from build123d import *

# Parameters (mm, degrees)
SKETCH1_W           = 22
SKETCH1_H           = 50
BOSS_EXTRUDE1_DEPTH = 4.25


with BuildPart() as part:
    # Sketch1 → Boss-Extrude1 (new body, symmetric)
    with BuildSketch(Plane.XY):
        with BuildLine():
            Line((-498.569276331, 84.968707483), (501.430723669, 84.968707483))
            Line((501.430723669, 84.968707483), (501.430723669, 62.328707483))
            ThreePointArc((501.430723669, 62.328707483), (498.250723669, 59.148707483), (501.430723669, 55.968707483))
            Line((501.430723669, 55.968707483), (551.430723669, 55.968707483))
            Line((551.430723669, 55.968707483), (551.430723669, -53.031292517))
            Line((551.430723669, -53.031292517), (501.430723669, -53.031292517))
            ThreePointArc((501.430723669, -53.031292517), (498.250723669, -56.211292517), (501.430723669, -59.391292517))
            Line((501.430723669, -59.391292517), (501.430723669, -82.031292517))
            Line((501.430723669, -82.031292517), (-498.569276331, -82.031292517))
            Line((-498.569276331, -82.031292517), (-498.569276331, -59.391292517))
            ThreePointArc((-498.569276331, -59.391292517), (-495.389276331, -56.211292517), (-498.569276331, -53.031292517))
            Line((-498.569276331, -53.031292517), (-548.569276331, -53.031292517))
            Line((-548.569276331, -53.031292517), (-548.569276331, 55.968707483))
            Line((-548.569276331, 55.968707483), (-498.569276331, 55.968707483))
            ThreePointArc((-498.569276331, 55.968707483), (-495.389276331, 59.148707483), (-498.569276331, 62.328707483))
            Line((-498.569276331, 62.328707483), (-498.569276331, 84.968707483))
        make_face()
        with Locations((520.430723669, 1.468707483)):
            Rectangle(SKETCH1_W, SKETCH1_H, mode=Mode.SUBTRACT)
        with Locations((-517.569276331, 1.468707483)):
            Rectangle(SKETCH1_W, SKETCH1_H, mode=Mode.SUBTRACT)
    extrude(amount=BOSS_EXTRUDE1_DEPTH, both=True)


solid = part.part
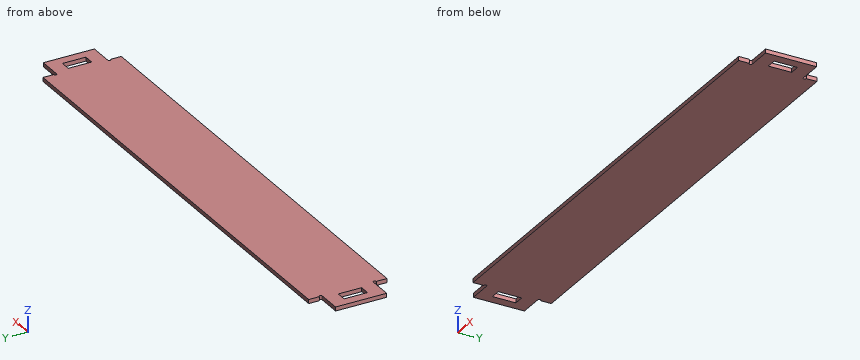
Work out the finished part from the listing and answer in its coordinate system (mm). Round coordinates to 2 decimals unless told otherwise and drop trailing zeros. Order: outer loops, then holes, each group sorted by start corner. A loop starts at its lowest first (then second) coordinate and runs counter-clockwise, first axis right, second up. Notation, with made-up numbers: M 21,50 L 38,50 A20 ccw 38,73 Z; hole C -25.75,83 d4. An arc over 180 degrees is marked long. Put each result on its own line as item: value. Start each with the question number.
Q1. Straight lines are drawn through the part: L1, parallel to X at y = 10, z = -0.5; L2, parallel to X at y = -64, z = 2.75; L3, parallel to X at y = 61, z = 1.5. For each, find the intervals that lie inside material, in ascending order. Write a range as [from, to].
Q2. Section A-A, the plane y = 4 is taken. Write down the section's boundary in (x, z).
Q3. Section B-B, the plane z = 1.5 is taken. Write down the section's boundary in (x, y).
Q4. Flat-ended cylindrical pins translate along their axes: pin 1 (2.5 mm diameter, centred on x = -534, z = -0.5, fed in from -Y); pin 2 (4 mm diameter, centred on y = -70, z = -2, fed in from -X); pin 3 (4 mm diameter, centred on y = -75.5, z = 2, fed in from +X). Find the tip coordinate at first contact, or state that the pin passes through.
Findings below:
1. L1: x = [-548.57, -528.57], [-506.57, 509.43], [531.43, 551.43]
1. L2: x = [-498.57, 501.43]
1. L3: x = [-495.98, 498.85]
2. outline: M -548.57,-4.25 L -528.57,-4.25 L -528.57,4.25 L -548.57,4.25 Z; M -506.57,-4.25 L 509.43,-4.25 L 509.43,4.25 L -506.57,4.25 Z; M 531.43,-4.25 L 551.43,-4.25 L 551.43,4.25 L 531.43,4.25 Z
3. outline: M -548.57,-53.03 L -498.57,-53.03 A3.18 cw -498.57,-59.39 L -498.57,-82.03 L 501.43,-82.03 L 501.43,-59.39 A3.18 cw 501.43,-53.03 L 551.43,-53.03 L 551.43,55.97 L 501.43,55.97 A3.18 cw 501.43,62.33 L 501.43,84.97 L -498.57,84.97 L -498.57,62.33 A3.18 cw -498.57,55.97 L -548.57,55.97 Z; hole M -528.57,-23.53 L -506.57,-23.53 L -506.57,26.47 L -528.57,26.47 Z; hole M 509.43,-23.53 L 531.43,-23.53 L 531.43,26.47 L 509.43,26.47 Z
4. pin 1: stops at y = -53.03
4. pin 2: stops at x = -498.57
4. pin 3: stops at x = 501.43
